Build history of the part. All positions in model axes, mm. Face numbers are marked on the shaded views. A direction names the side the tool comes from. Coordinates: 2 decimals unless noted, no trailing zeros. Loops run counter-clockwise (first coordinate to the right, second up) from the corner with the lowest first, then second, coordinate; pieces in that order, holes last.
Item 1: Cut at A-A (z = 6). List the corners of the cut face in (x, y), and give its area (3 significant figures).
Item 2: Drill centre lines: line 1 along Z through (x, y) = (-7.25, -0.25); line 2 along Z through (x, y) = (-3.25, -6); line 3 along Z through (x, y) = (5, 3). Where is each one in solid material? Low to high.
Item 3: Flat gauge pins, fed straight in: pin 1 (6 mm diameter, centred on x = -4, z = 70.5, fed in from +Y); pin 2 (2.5 mm diameter, centred on x = 1, y = 0, fed in from +Z); pin 3 (3 mm diameter, centred on y = 0, z = 6, fed in from +X) (3 decimals); pin 4 (10 mm diameter, centred on x = -2.5, z = 81.5, fed in from -Y). Where does each tip first touch, or does it go through?
Item 4: Cut at C-C (z = 107). List the corners of the cut face in (x, y), and give its area (3 significant figures).
Item 5: 3-axis set-ups, long thin cutter, end or side, ignore diameter. For the marked faces 1, 2 and 3: which of +Z, -Z, +X, -X, +Y, -Y reach the whole face in a straight line?
Item 6: Cut at B-B (y = 0). Count the separate pieces of the cut face and the enclosed holes in it, and give its area (3 significant figures).
Item 7: Cut at D-D (x = 6.5). List the corners of the cut face in (y, z).
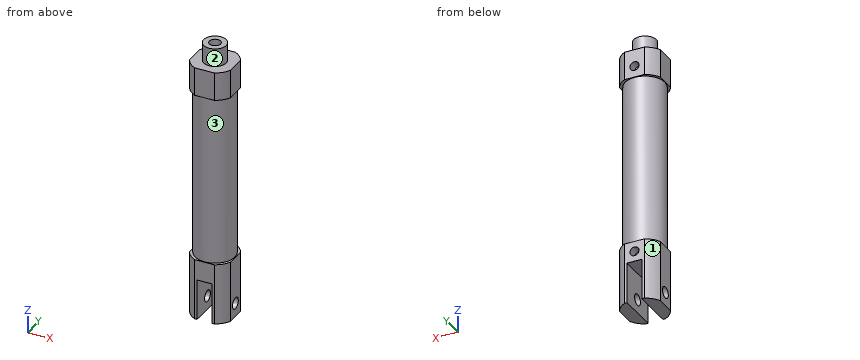
from build123d import *

# Parameters (mm, degrees)
BOSS_EXTRUDE1_DEPTH = 27
SKETCH2_R           = 8.75
BOSS_EXTRUDE2_DEPTH = 75
BOSS_EXTRUDE3_DEPTH = 12.5
SKETCH4_R           = 5
BOSS_EXTRUDE4_DEPTH = 8
SKETCH5_R           = 2.5
CUT_EXTRUDE1_DEPTH  = 50
SKETCH6_R           = 2
CUT_EXTRUDE2_DEPTH  = 4
CUT_EXTRUDE4_DEPTH  = 125.142055726
SKETCH10_R          = 2
CUT_EXTRUDE5_DEPTH  = 4
SKETCH11_R          = 2.5
CUT_EXTRUDE6_DEPTH  = 125.142055726


with BuildPart() as part:
    # Sketch1 → Boss-Extrude1 (new body)
    with BuildSketch(Plane.XY):
        with BuildLine():
            Line((-4.358898944, -9), (4.358898944, -9))
            ThreePointArc((4.358898944, -9), (7.071067812, -7.071067812), (9, -4.358898944))
            Line((9, -4.358898944), (9, 4.358898944))
            ThreePointArc((9, 4.358898944), (7.071067812, 7.071067812), (4.358898944, 9))
            Line((4.358898944, 9), (-4.358898944, 9))
            ThreePointArc((-4.358898944, 9), (-7.071067812, 7.071067812), (-9, 4.358898944))
            Line((-9, 4.358898944), (-9, -4.358898944))
            ThreePointArc((-9, -4.358898944), (-7.071067812, -7.071067812), (-4.358898944, -9))
        make_face()
    extrude(amount=BOSS_EXTRUDE1_DEPTH)

    # Sketch2 → Boss-Extrude2 (add)
    with BuildSketch(Plane.XY.offset(27)):
        Circle(SKETCH2_R)
    extrude(amount=BOSS_EXTRUDE2_DEPTH)

    # Sketch3 → Boss-Extrude3 (add)
    with BuildSketch(Plane.XY.offset(102)):
        with BuildLine():
            Line((-4.358898944, -9), (4.358898944, -9))
            ThreePointArc((4.358898944, -9), (7.071067812, -7.071067812), (9, -4.358898944))
            Line((9, -4.358898944), (9, 4.358898944))
            ThreePointArc((9, 4.358898944), (7.071067812, 7.071067812), (4.358898944, 9))
            Line((4.358898944, 9), (-4.358898944, 9))
            ThreePointArc((-4.358898944, 9), (-7.071067812, 7.071067812), (-9, 4.358898944))
            Line((-9, 4.358898944), (-9, -4.358898944))
            ThreePointArc((-9, -4.358898944), (-7.071067812, -7.071067812), (-4.358898944, -9))
        make_face()
    extrude(amount=BOSS_EXTRUDE3_DEPTH)

    # Sketch4 → Boss-Extrude4 (add)
    with BuildSketch(Plane.XY.offset(114.5)):
        Circle(SKETCH4_R)
    extrude(amount=BOSS_EXTRUDE4_DEPTH)

    # Sketch5 → Cut-Extrude1 (cut)
    with BuildSketch(Plane.XY.offset(122.5)):
        Circle(SKETCH5_R)
    extrude(amount=-CUT_EXTRUDE1_DEPTH, mode=Mode.SUBTRACT)

    # Sketch6 → Cut-Extrude2 (cut)
    with BuildSketch(Plane(origin=(0, 9, 0), x_dir=(1, 0, 0), z_dir=(0, 1, 0))):
        with Locations(Location((0, -107, 0), (0, 0, 270))):
            Circle(SKETCH6_R)
    extrude(amount=-CUT_EXTRUDE2_DEPTH, mode=Mode.SUBTRACT)

    # Sketch9 → Cut-Extrude4 (cut, through all)
    with BuildSketch(Plane(origin=(0, 9, 0), x_dir=(1, 0, 0), z_dir=(0, 1, 0))):
        Polygon((3.3, 0), (0, 0), (-3.3, 0), (-3.3, -18), (3.3, -18), align=None)
    extrude(amount=-CUT_EXTRUDE4_DEPTH, mode=Mode.SUBTRACT)

    # Sketch10 → Cut-Extrude5 (cut)
    with BuildSketch(Plane(origin=(0, 9, 0), x_dir=(1, 0, 0), z_dir=(0, 1, 0))):
        with Locations(Location((0, -22.5, 0), (0, 0, 180))):
            Circle(SKETCH10_R)
    extrude(amount=-CUT_EXTRUDE5_DEPTH, mode=Mode.SUBTRACT)

    # Sketch11 → Cut-Extrude6 (cut, through all)
    with BuildSketch(Plane.ZY.offset(9)):
        with Locations((6, 0)):
            Circle(SKETCH11_R)
    extrude(amount=-CUT_EXTRUDE6_DEPTH, mode=Mode.SUBTRACT)


solid = part.part
Filled sheet:
1. outline: (-9, -4.36) arc R10 ccw to (-4.36, -9) - (-3.3, -9) - (-3.3, -2.5) - (-9, -2.5) - close; (-9, 2.5) - (-3.3, 2.5) - (-3.3, 9) - (-4.36, 9) arc R10 ccw to (-9, 4.36) - close; (3.3, -9) - (4.36, -9) arc R10 ccw to (9, -4.36) - (9, -2.5) - (3.3, -2.5) - close; (3.3, 2.5) - (9, 2.5) - (9, 4.36) arc R10 ccw to (4.36, 9) - (3.3, 9) - close
1. area: 115 mm2
2. line 1: z = 0 to 3.51, 8.49 to 114.5
2. line 2: z = 18 to 114.5
2. line 3: z = 0 to 114.5
3. pin 1: stops at y = 8.69
3. pin 2: stops at z = 72.5
3. pin 3: passes through
3. pin 4: stops at y = -8.75
4. outline: (-9, -4.36) arc R10 ccw to (-4.36, -9) - (4.36, -9) arc R10 ccw to (9, -4.36) - (9, 4.36) arc R10 ccw to (4.36, 9) - (2, 9) - (2, 5) - (-2, 5) - (-2, 9) - (-4.36, 9) arc R10 ccw to (-9, 4.36) - close; hole circle Ø5 at (0, 0)
4. area: 255 mm2
5. face 1: +Z, -Z, -X, +Y
5. face 2: +Z
5. face 3: none
6. separate pieces: 3
6. enclosed holes: 0
6. area: 1,680 mm2
7. outline: (-7.6, 0) - (7.6, 0) - (7.6, 27) - (5.86, 27) - (5.86, 102) - (7.6, 102) - (7.6, 114.5) - (-7.6, 114.5) - (-7.6, 102) - (-5.86, 102) - (-5.86, 27) - (-7.6, 27) - close; hole circle Ø5 at (0, 6)
